```python
from build123d import *

# Parameters (mm, degrees)
BOSS_EXTRUDE1_DEPTH            = 20
CUT_EXTRUDE4_REACH             = 41.693
SKETCH2_R                      = 2
CUT_EXTRUDE4_DIRECTION_2_DEPTH = 40.693324376
CUT_EXTRUDE5_REACH             = 47.651
SKETCH3_R                      = 2


with BuildPart() as part:
    # Sketch1 → Boss-Extrude1 (new body)
    with BuildSketch(Plane(origin=(0, 0, 0), x_dir=(1, 0, 0), z_dir=(0, 1, 0))):
        Polygon((0, 13.4), (0, -14.52), (-28, -14.52), (-28, -16.6), (2, -16.6), (2, 13.4), align=None)
    extrude(amount=BOSS_EXTRUDE1_DEPTH)

    # Sketch2 → Cut-Extrude4 (cut, up to next)
    with BuildSketch(Plane(origin=(2, 0, 0), x_dir=(0, 0, -1), z_dir=(1, 0, 0)), mode=Mode.PRIVATE) as cut_extrude4_sk1:
        with Locations(Location((0, 15, 0), (0, 0, 180))):
            Circle(SKETCH2_R)
    cut_extrude4_tool1 = extrude(cut_extrude4_sk1.sketch, amount=-CUT_EXTRUDE4_REACH, mode=Mode.PRIVATE) & part.part
    # Sketch2 → Cut-Extrude4 (cut, up to next)
    with BuildSketch(Plane(origin=(2, 0, 0), x_dir=(0, 0, -1), z_dir=(1, 0, 0)), mode=Mode.PRIVATE) as cut_extrude4_sk2:
        with Locations(Location((0, 5, 0), (0, 0, 180))):
            Circle(SKETCH2_R)
    cut_extrude4_tool2 = extrude(cut_extrude4_sk2.sketch, amount=-CUT_EXTRUDE4_REACH, mode=Mode.PRIVATE) & part.part
    add(cut_extrude4_tool1.solids().sort_by_distance((2, 15, 0))[0], mode=Mode.SUBTRACT)
    add(cut_extrude4_tool2.solids().sort_by_distance((2, 5, 0))[0], mode=Mode.SUBTRACT)

    # Sketch2 → Cut-Extrude4 direction 2 (cut)
    with BuildSketch(Plane(origin=(2, 0, 0), x_dir=(0, 0, -1), z_dir=(1, 0, 0))):
        with Locations(Location((0, 15, 0), (0, 0, 180))):
            Circle(SKETCH2_R)
        with Locations(Location((0, 5, 0), (0, 0, 180))):
            Circle(SKETCH2_R)
    extrude(amount=CUT_EXTRUDE4_DIRECTION_2_DEPTH, mode=Mode.SUBTRACT)

    # Sketch3 → Cut-Extrude5 (cut, up to next)
    with BuildSketch(Plane.XY.offset(16.6), mode=Mode.PRIVATE) as cut_extrude5_sk1:
        with Locations((-10.523881442, 15)):
            Circle(SKETCH3_R)
    cut_extrude5_tool1 = extrude(cut_extrude5_sk1.sketch, amount=-CUT_EXTRUDE5_REACH, mode=Mode.PRIVATE) & part.part
    # Sketch3 → Cut-Extrude5 (cut, up to next)
    with BuildSketch(Plane.XY.offset(16.6), mode=Mode.PRIVATE) as cut_extrude5_sk2:
        with Locations((-10.523881442, 5)):
            Circle(SKETCH3_R)
    cut_extrude5_tool2 = extrude(cut_extrude5_sk2.sketch, amount=-CUT_EXTRUDE5_REACH, mode=Mode.PRIVATE) & part.part
    add(cut_extrude5_tool1.solids().sort_by_distance((-10.523881, 15, 16.6))[0], mode=Mode.SUBTRACT)
    add(cut_extrude5_tool2.solids().sort_by_distance((-10.523881, 5, 16.6))[0], mode=Mode.SUBTRACT)


solid = part.part
```
CAD build for the part. Positions are in the model's coordinates, mm. A direction names the side the tool comes from. Round coordinates to 2 decimals unless told otherwise and drop trailing zeros. Order: outer loops, then holes, each group sorted by start corner. A loop starts at its lowest first (then second) coordinate and runs counter-clockwise, first axis right, second up. Notation, with made-up numbers: (70.25, -34) - (100.25, -34) arc R15 cw to (100.25, -23) - close; hole circle Ø7 at (-39.5, 47). An arc over 180 degrees is marked (long way). Answer as CSV lines item,"result". Start each with the question number.
1. Pin check, flat tips, straight feed: pin 1 (2 mm diameter, centred on y = 12.5, z = 7, fed in from -X); pin 2 (6 mm diameter, centred on x = -11, y = 11.5, fed in from -Z); pin 3 (3.5 mm diameter, centred on x = -10.52, y = 15, fed in from +Z). Stop position of each tip, or through.
2. Tool access for faces 4 (the face through (-14, 10, 14.52)), 5 (the face through (-6, 0, 15)): list every direction of +Z, -Z, +X, -X, +Y, -Y with a clear straight run to the whole face (end or side of a thin tool).
3. Drill centre lines: L1, parallel to Y at x = 1.3, z = 0; L2, parallel to Z at x = 0.55, y = 5; L3, parallel to Z at x = -7.25, y = 3. Where is each one in solid material? Low to high. Write a range as [from, to].
4. Saw through at B-B, the plane z = 0. Write the cut outline in (x, y).
5. Saw through at D-D, the plane y = 12. Write the cut outline in (x, z), and give its area (3 significant figures).
6. Saw through at C-C, the plane x = -11.75. Write the cut outline in (y, z), and give its area (3 significant figures).
7. Saw through at A-A, the plane y = 5. Write the cut outline in (x, z).
8. Pull direction Z, two halves, no side cores. Call faces 1 (the face through (-8.616, 5.601, 15.575)), 2 (the face through (1, 10, -13.4)), 3 (the face through (1, 7, 0)): +Z half, -Z half, draft (parallel to the pull), parting line (faces both ways), or undercut.
Model answer:
1,pin 1,"stops at x = 0"
1,pin 2,"stops at z = 14.52"
1,pin 3,"passes through"
2,face 4,"-Z, -X, +Y, -Y"
2,face 5,"+Z, -Z, +X, -X, -Y"
3,L1,"y = [0, 3], [7, 13], [17, 20]"
3,L2,"z = [-13.4, -2], [2, 16.6]"
3,L3,"z = [14.52, 16.6]"
4,outline,"(0, 0) - (2, 0) - (2, 3) - (0, 3) - close; (0, 7) - (2, 7) - (2, 13) - (0, 13) - close; (0, 17) - (2, 17) - (2, 20) - (0, 20) - close"
5,outline,"(-28, 14.52) - (0, 14.52) - (0, -13.4) - (2, -13.4) - (2, 16.6) - (-28, 16.6) - close"
5,area,"118 mm²"
6,outline,"(0, 14.52) - (3.42, 14.52) - (3.42, 16.6) - (0, 16.6) - close; (6.58, 14.52) - (13.42, 14.52) - (13.42, 16.6) - (6.58, 16.6) - close; (16.58, 14.52) - (20, 14.52) - (20, 16.6) - (16.58, 16.6) - close"
6,area,"28.5 mm²"
7,outline,"(-28, 14.52) - (-12.52, 14.52) - (-12.52, 16.6) - (-28, 16.6) - close; (-8.52, 14.52) - (0, 14.52) - (0, 2) - (2, 2) - (2, 16.6) - (-8.52, 16.6) - close; (0, -13.4) - (2, -13.4) - (2, -2) - (0, -2) - close"
8,face 1,"draft"
8,face 2,"-Z half"
8,face 3,"undercut"
